Design review of the part built by this model. Coordinates are the model's own, in mm. A direction names the side the tool comes from. Round coordinates to 2 decimals unless told otherwise and drop trailing zeros. Loops run counter-clockwise (first coordinate to the right, second up) from the corner with the lowest first, then second, coordinate; pieces in that order, holes last. Notation, with made-up numbers: M -27.5,-27.75 L 7.5,-27.75 A22 ccw 7.5,-21.75 Z; hole C -12.5,33 d4. An arc over 180 degrees is marked long. Use a Markdown table: item, result.
from build123d import *

# Parameters (mm, degrees)
SKETCH_1_W          = 30
SKETCH_1_H          = 30
SKETCH_1_R          = 0.65
SKETCH_1_R_2        = 4
SKETCH_1_R_3        = 1.4
EXTRUDE_1_DEPTH     = 2
SKETCH_2_R          = 2.1
SKETCH_2_R_2        = 1.3
EXTRUDE_3_DEPTH     = 2
CUT_EXTRUDE_START   = -2
SKETCH_2_6_R        = 1.3
SKETCH_2_6_R_2      = 1.4
SKETCH_2_6_R_3      = 2.1
CUT_EXTRUDE_2_DEPTH = 2


with BuildPart() as part:
    # 草图1 → 凸台-拉伸1 (new body)
    with BuildSketch(Plane(origin=(0, 0, 0), x_dir=(1, 0, 0), z_dir=(0, 1, 0))):
        Rectangle(SKETCH_1_W, SKETCH_1_H)
        with Locations(Location((8, 0, 0), (0, 0, 270))):
            Circle(SKETCH_1_R, mode=Mode.SUBTRACT)
        with Locations(Location((0, -8, 0), (0, 0, 270))):
            Circle(SKETCH_1_R, mode=Mode.SUBTRACT)
        with Locations(Location((-8, 0, 0), (0, 0, 270))):
            Circle(SKETCH_1_R, mode=Mode.SUBTRACT)
        with Locations(Location((0, 8, 0), (0, 0, 270))):
            Circle(SKETCH_1_R, mode=Mode.SUBTRACT)
        with Locations(Location((0, 0, 0), (0, 0, 270))):
            Circle(SKETCH_1_R_2, mode=Mode.SUBTRACT)
        with Locations(Location((12, 12, 0), (0, 0, 270))):
            Circle(SKETCH_1_R_3, mode=Mode.SUBTRACT)
        with Locations(Location((-12, 12, 0), (0, 0, 270))):
            Circle(SKETCH_1_R_3, mode=Mode.SUBTRACT)
        with Locations(Location((12, -12, 0), (0, 0, 270))):
            Circle(SKETCH_1_R_3, mode=Mode.SUBTRACT)
        with Locations(Location((-12, -12, 0), (0, 0, 270))):
            Circle(SKETCH_1_R_3, mode=Mode.SUBTRACT)
    extrude(amount=EXTRUDE_1_DEPTH)

    # 草图2 → 凸台-拉伸3 (add)
    # profile 1 of 3: a face of its own
    with BuildSketch(Plane(origin=(0, 2, 0), x_dir=(1, 0, 0), z_dir=(0, 1, 0))):
        with Locations(Location((-7, -7, 0), (0, 0, 270))):
            Circle(SKETCH_2_R)
        with Locations(Location((-7, -7, 0), (0, 0, 270))):
            Circle(SKETCH_2_R_2, mode=Mode.SUBTRACT)
    # profile 2 of 3: a face of its own
    with BuildSketch(Plane(origin=(0, 2, 0), x_dir=(1, 0, 0), z_dir=(0, 1, 0))):
        with Locations(Location((-7, 7, 0), (0, 0, 270))):
            Circle(SKETCH_2_R)
        with Locations(Location((-7, 7, 0), (0, 0, 270))):
            Circle(SKETCH_2_R_2, mode=Mode.SUBTRACT)
    # profile 3 of 3: a face of its own
    with BuildSketch(Plane(origin=(0, 2, 0), x_dir=(1, 0, 0), z_dir=(0, 1, 0))):
        with Locations(Location((7, 7, 0), (0, 0, 270))):
            Circle(SKETCH_2_R)
        with Locations(Location((7, 7, 0), (0, 0, 270))):
            Circle(SKETCH_2_R_2, mode=Mode.SUBTRACT)
    extrude(amount=EXTRUDE_3_DEPTH)

    # 草图2<6> → 切除-拉伸2 (cut)
    # profile 1 of 6: a face of its own
    with BuildSketch(Plane(origin=(0, 2, 0), x_dir=(1, 0, 0), z_dir=(0, 1, 0)).offset(CUT_EXTRUDE_START)):
        with Locations(Location((-7, 7, 0), (0, 0, 270))):
            Circle(SKETCH_2_6_R)
    # profile 2 of 6: a face of its own
    with BuildSketch(Plane(origin=(0, 2, 0), x_dir=(1, 0, 0), z_dir=(0, 1, 0)).offset(CUT_EXTRUDE_START)):
        with Locations(Location((-7, -7, 0), (0, 0, 270))):
            Circle(SKETCH_2_6_R)
    # profile 3 of 6: a face of its own
    with BuildSketch(Plane(origin=(0, 2, 0), x_dir=(1, 0, 0), z_dir=(0, 1, 0)).offset(CUT_EXTRUDE_START)):
        with Locations(Location((7, 7, 0), (0, 0, 270))):
            Circle(SKETCH_2_6_R)
    # profile 4 of 6: a face of its own
    with BuildSketch(Plane(origin=(0, 2, 0), x_dir=(1, 0, 0), z_dir=(0, 1, 0)).offset(CUT_EXTRUDE_START)):
        with BuildLine():
            Line((15, -10.757359313), (5.795554958, -1.552914271))
            ThreePointArc((5.795554958, -1.552914271), (4.242640687, -4.242640687), (1.552914271, -5.795554958))
            Line((1.552914271, -5.795554958), (10.757359313, -15))
            Line((10.757359313, -15), (15, -15))
            Line((15, -15), (15, -10.757359313))
        make_face()
        with Locations((12, -12)):
            Circle(SKETCH_2_6_R_2, mode=Mode.SUBTRACT)
        with Locations((7, -7)):
            Circle(SKETCH_2_6_R_3, mode=Mode.SUBTRACT)
    # profile 5 of 6: a face of its own
    with BuildSketch(Plane(origin=(0, 2, 0), x_dir=(1, 0, 0), z_dir=(0, 1, 0)).offset(CUT_EXTRUDE_START)):
        with Locations((7, -7)):
            Circle(SKETCH_2_6_R_3)
        with Locations((7, -7)):
            Circle(SKETCH_2_6_R, mode=Mode.SUBTRACT)
    # profile 6 of 6: a face of its own
    with BuildSketch(Plane(origin=(0, 2, 0), x_dir=(1, 0, 0), z_dir=(0, 1, 0)).offset(CUT_EXTRUDE_START)):
        with Locations((7, -7)):
            Circle(SKETCH_2_6_R)
    extrude(amount=CUT_EXTRUDE_2_DEPTH, mode=Mode.SUBTRACT)


solid = part.part
1. The part is to be moulded in two halves that separate along Z. For faces 1 (the face through (5.6, 4, -6.6)), 2 (the face through (12.95, 0.99, -13.03)), 3 (the face through (-2, 1, 15)), say which applies: pulls with the +Z half, pulls with the -Z half, needs draft (parallel to the pull), parting line crosses it, or undercut.
Check values:
| item | result |
|---|---|
| face 1 | needs draft |
| face 2 | undercut |
| face 3 | pulls with the +Z half |
2. Take a section at A-A on x = -12. Give the boundary of the cut face in (y, z).
Check values:
| item | result |
|---|---|
| outline | M 0,-15 L 2,-15 L 2,-13.4 L 0,-13.4 Z; M 0,-10.6 L 2,-10.6 L 2,10.6 L 0,10.6 Z; M 0,13.4 L 2,13.4 L 2,15 L 0,15 Z |
3. Take a section at C-C on z = -12. Give the boundary of the cut face in (x, y).
Check values:
| item | result |
|---|---|
| outline | M -15,0 L -13.4,0 L -13.4,2 L -15,2 Z; M -10.6,0 L 10.6,0 L 10.6,2 L -10.6,2 Z; M 13.4,0 L 15,0 L 15,2 L 13.4,2 Z |
4. Machinability: for faces 4 (the face through (-8.4, 4, 7.4)), 5 (the face through (-4.918, 2.986, 6.727)), 6 (the face through (10.46, 0.99, 6.22)), which of the approach directions +Z, -Z, +X, -X, +Y, -Y give a long, thin tool a straight path to every point of the face, cutting with its end or side? Answer none if there is none.
Check values:
| item | result |
|---|---|
| face 4 | +Z, -Z, +X, -X, +Y |
| face 5 | +Y |
| face 6 | +Y, -Y |
5. Insertion check: pin 1 (2 mm diameter, centred on x = -8, z = 0, fed in from -Y); pin 2 (3.5 mm diameter, centred on x = 12, z = -12, fed in from +Y). Each pin has a flat end and moves straight along its axis. Give the tip position at first contact, or say it passes through.
Check values:
| item | result |
|---|---|
| pin 1 | stops at y = 0 |
| pin 2 | stops at y = 2 |
6. Take a section at B-B on y = 3.4. Give the boundary of the cut face in (x, z).
Check values:
| item | result |
|---|---|
| outline | C -7,-7 d4.2; C -7,7 d4.2; C 7,-7 d4.2; hole C -7,-7 d2.6; hole C -7,7 d2.6; hole C 7,-7 d2.6 |
7. Wall thickness on line 1 along X through (y, z) = (2.5, -7); line 2 along X through (y, z) = (1.05, -12); line 3 along Z through (x, y) = (-7.25, 1.4): over which ranges is each line inside the solid? List them lowest first. Write a range as from..to.
Check values:
| item | result |
|---|---|
| line 1 | x = -9.1..-8.3, -5.7..-4.9, 4.9..5.7, 8.3..9.1 |
| line 2 | x = -15..-13.4, -10.6..10.6, 13.4..15 |
| line 3 | z = -15..-8.28, -5.72..5.72, 8.28..15 |
8. Take a section at D-D on y = 0.7. Count the separate pieces of the cut face and the enclosed holes in it, and give its area (3 significant figures).
Check values:
| item | result |
|---|---|
| separate pieces | 1 |
| enclosed holes | 11 |
| area | 726 mm² |
